Here's the drawing with two shaded views (mm, measured from the low corner). I have some questions. A direction names the side the tool comes from. Give positions to 0.01 mm unless a question says otherwise; leave off trailing zeros. Loops run counter-clockwise (first coordinate to the right, second up) from the corner with the lowest first, then second, coordinate; pieces in that order, holes last.
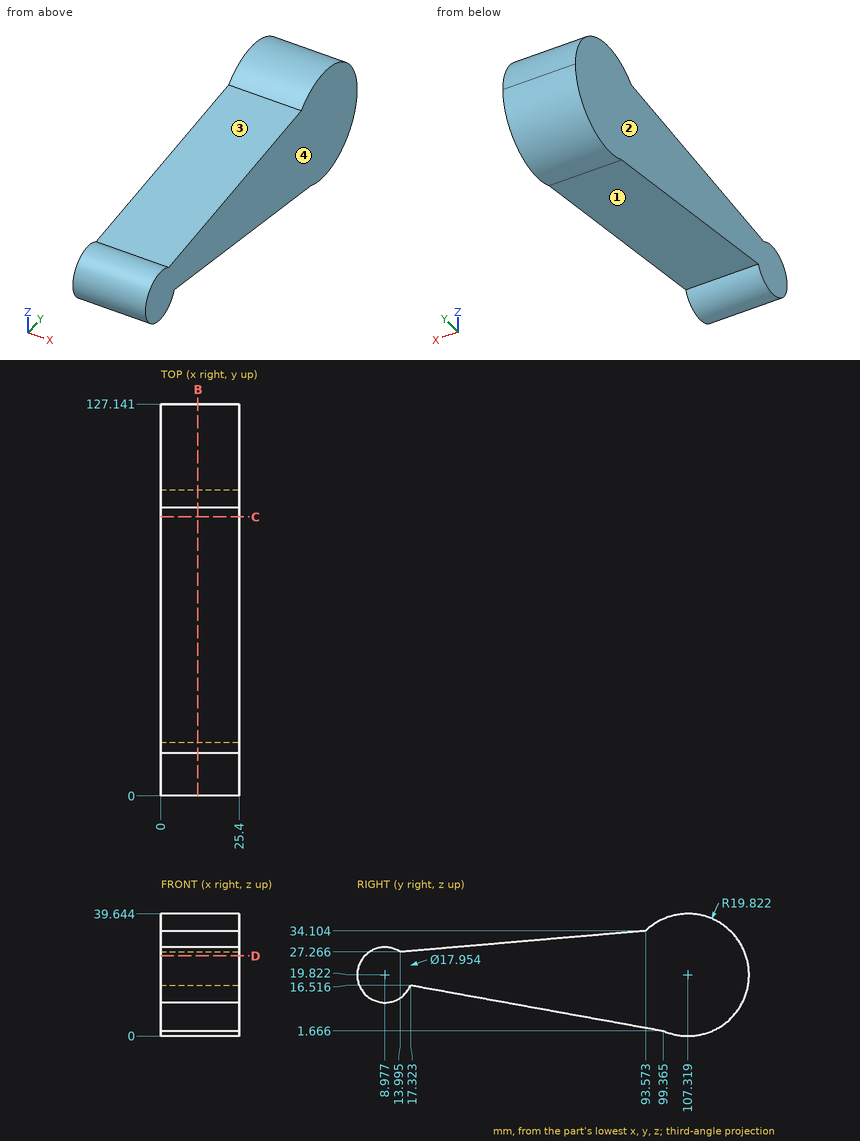
(1) Please list where these lines run through material, in increasing order: probe 1 along Y at (x, z) = (2.75, 17.5) (1 decimal); probe 2 along Z at (x, y) = (18.25, 114) (1 decimal); probe 3 along Z at (x, y) = (2, 55.5) (1 decimal).
Returned:
probe 1: y = 0.3 to 127
probe 2: z = 1.2 to 38.5
probe 3: z = 9.6 to 30.8
(2) Will these pins go through, and if not, where does the flat tip stop? P1, Ø8, axis at x = 14, y = 76.5, coming from the +Z side; P2, Ø12, axis at x = 5.5, y = 102.5, coming from the +Z side; P3, Ø4, axis at x = 9, z = 15.5, coming from the +Y side (1 decimal); P4, Ø2, axis at x = 19.5, z = 31, coming from the +Y side.
Returned:
P1: stops at z = 32.98
P2: stops at z = 39.64
P3: stops at y = 127
P4: stops at y = 124.33
(3) Suppose I cut it at B-B on x = 12. List the corners of the cut face in (y, z) for me (1 decimal), plus the area to 4 significant figures.
Returned:
outline: (14, 27.3) arc R9 ccw (long way) to (17.3, 16.5) - (99.4, 1.7) arc R19.8 ccw (long way) to (93.6, 34.1) - close
area: 2,995 mm2
(4) Thinking about a two-plate mould opening in Y: for the marked faces 3 and 4, which applies, pulls with the +Y half, pulls with the -Y half, needs draft (parallel to the pull), parting line crosses it, or undercut?
Returned:
face 3: undercut
face 4: needs draft
(5) Suppose I cut it at C-C on y = 90.5. List the corners of the cut face in (x, z) for me.
Returned:
outline: (0, 3.27) - (25.4, 3.27) - (25.4, 33.84) - (0, 33.84) - close
(6) Which directions (+Z, -Z, +X, -X, +Y, -Y) give clear straight access to the entire face, cutting with the end or side of a thin tool? Please do the marked faces 1 and 2.
Returned:
face 1: -Z, +X, -X
face 2: +Z, -Z, -X, +Y, -Y
(7) Suppose I cut it at D-D on z = 26. List the corners of the cut face in (x, y) for me.
Returned:
outline: (0, 2.46) - (25.4, 2.46) - (25.4, 126.15) - (0, 126.15) - close
